from build123d import *

# Parameters (mm, degrees)
F0_R     = 7.4
F1_DEPTH = 20
F2_R     = 6
F2_R_2   = 4
F3_DEPTH = 15


with BuildPart() as f1:
    # F0 (on Front) → F1 (new body)
    with BuildSketch(Plane.XZ):
        Circle(F0_R)
    extrude(amount=-F1_DEPTH)

    # F2 (on face) → F3 (cut)
    with BuildSketch(Plane.XZ):
        Circle(F2_R)
        Circle(F2_R_2, mode=Mode.SUBTRACT)
    extrude(amount=-F3_DEPTH, mode=Mode.SUBTRACT)


solid = f1.part
The model under review builds one solid part; all positions refer to its coordinate system, in mm. A direction names the side the tool comes from. Round coordinates to 2 decimals unless told otherwise and drop trailing zeros. Order: outer loops, then holes, each group sorted by start corner. A loop starts at its lowest first (then second) coordinate and runs counter-clockwise, first axis right, second up. Notation, with made-up numbers: (-20, 13.25) - (1, 13.25) arc R18 cw to (1, 33.25) - close; hole circle Ø11 at (63, 11). An arc over 180 degrees is marked (long way). Use one line per item in the form item = value.
Q1. Clearance check with flat-ended pins moving along their axes: P1, Ø3, axis at x = -5, y = 15, coming from the -Z side; P2, Ø4, axis at x = -3, y = 8, coming from the +Z side; P3, Ø4, axis at y = 7, z = -2.5, coming from the +X side. State where each tip first meets the part, or that it passes through.
Response values:
P1 = -6.52
P2 = 7.33
P3 = 7.38
Q2. Add section B-B on x = 0. Give the boundary of the cut face in (y, z), then the cut area to 3 significant figures.
Response values:
outline = (0, -7.4) - (20, -7.4) - (20, 7.4) - (0, 7.4) - (0, 6) - (15, 6) - (15, 4) - (0, 4) - (0, -4) - (15, -4) - (15, -6) - (0, -6) - close
area = 236 mm^2
Q3. Mouldability with a two-part tool opening along Z and no side actions: class faces 3 (the flat face through (-1.42, 15, -3.92)), 4 (the flat face through (-1.1, 0, 6.1)), 5 (the cylindrical face through (-1.604, 9.86, -7.224)), 6 (the cylindrical face through (-6, 7, 0)) as pulls with the +Z half, pulls with the -Z half, needs draft (parallel to the pull), parting line crosses it, or undercut.
Response values:
face_3 = undercut
face_4 = needs draft
face_5 = parting line crosses it
face_6 = undercut
Q4. Add section D-D on x = 5.5. Give the boundary of the cut face in (y, z), then the cut area to 3 significant figures.
Response values:
outline = (0, -4.95) - (20, -4.95) - (20, 4.95) - (0, 4.95) - (0, 2.4) - (15, 2.4) - (15, -2.4) - (0, -2.4) - close
area = 126 mm^2
Q5. To check wall thickness, follow line 1 (Z direction, x = 0, y = 11.75); line 2 (X direction, y = 8.75, z = 3.25); line 3 (X direction, y = 12, z = -2). State the ranges of each line that lie inside material, in increasing order.
Response values:
line_1 = -7.4 to -6, -4 to 4, 6 to 7.4
line_2 = -6.65 to -5.04, -2.33 to 2.33, 5.04 to 6.65
line_3 = -7.12 to -5.66, -3.46 to 3.46, 5.66 to 7.12
Q6. Add section A-A on y = 4.25. Give the boundary of the cut face in (x, z).
Response values:
outline = circle Ø14.8 at (0, 0); circle Ø8 at (0, 0); hole circle Ø12 at (0, 0)
Q7. Tool access review of faces 1 (the cylindrical face through (-0.867, 7.395, -3.905)), 2 (the flat face through (0, 20, 0)): name each direction out of +Z, -Z, +X, -X, +Y, -Y from which nothing blocks a thin tool from reaching the whole face with its end or side.
Response values:
face_1 = -Y
face_2 = +Z, -Z, +X, -X, +Y
Q8. Add section C-C on z = 0. Give the boundary of the cut face in (x, y).
Response values:
outline = (-7.4, 0) - (-6, 0) - (-6, 15) - (-4, 15) - (-4, 0) - (4, 0) - (4, 15) - (6, 15) - (6, 0) - (7.4, 0) - (7.4, 20) - (-7.4, 20) - close
